Verification items for the finished model (mm, model axes). A direction names the side the tool comes from. Give positions to 0.01 mm unless a question says otherwise; leave off trailing zeros. Loops run counter-clockwise (first coordinate to the right, second up) from the corner with the lowest first, then second, coordinate; pieces in that order, holes last. Notation, with made-up numbers: M -25,4.5 L 14,4.5 A28 cw 14,43.5 Z; hole C 88,3.25 d11. An arc over 180 degrees is marked long. Use a Markdown table: item, result.
from build123d import *

# Parameters (mm, degrees)
BOSS_EXTRUDE1_DEPTH = 6.625
CUT_EXTRUDE1_DEPTH  = 13.25
SKETCH3_R           = 0.3
BOSS_EXTRUDE2_DEPTH = 4


with BuildPart() as part:
    # Sketch1 → Boss-Extrude1 (new, symmetric)
    with BuildSketch(Plane(origin=(0, 0, 0), x_dir=(0, 0, -1), z_dir=(1, 0, 0))):
        Polygon((0, 0), (0, 12.53), (14.54, 12.53), (18.15, 5), (18.15, 0), align=None)
    extrude(amount=BOSS_EXTRUDE1_DEPTH, both=True)

    # Sketch2 → Cut-Extrude1 (cut)
    with BuildSketch(Plane.XY):
        Polygon((-2.758412662, 1.863268477), (-2.758412662, 0.55), (2.758412662, 0.55), (2.758412662, 1.863268477), (3.967697722, 1.863268477), (3.967697722, 3.689249531), (5.425, 3.689249531), (5.425, 11.073209492), (3.069315997, 11.073209492), (3.069315997, 11.97), (-3.069315997, 11.97), (-3.069315997, 11.073209492), (-5.425, 11.073209492), (-5.425, 3.689249531), (-3.967697722, 3.689249531), (-3.967697722, 1.863268477), align=None)
    extrude(amount=-CUT_EXTRUDE1_DEPTH, mode=Mode.SUBTRACT)

    # Sketch3 → Boss-Extrude2 (add)
    with BuildSketch(Plane.XZ):
        with Locations(Location((2.54, -16.9, 0), (0, 0, 270))):
            Circle(SKETCH3_R)
        with Locations(Location((0, -16.9, 0), (0, 0, 270))):
            Circle(SKETCH3_R)
        with Locations(Location((-2.54, -16.9, 0), (0, 0, 270))):
            Circle(SKETCH3_R)
        with Locations(Location((0, -14.36, 0), (0, 0, 270))):
            Circle(SKETCH3_R)
        with Locations(Location((-2.54, -14.36, 0), (0, 0, 270))):
            Circle(SKETCH3_R)
        with Locations(Location((2.54, -14.36, 0), (0, 0, 270))):
            Circle(SKETCH3_R)
    extrude(amount=BOSS_EXTRUDE2_DEPTH)


solid = part.part
(1) Draft check along Y on faces 3 (the flat face through (6.625, 6, -9)), 4 (the flat face through (0, 12.53, -7)), 5 (the flat face through (-3.968, 3, -7)). Enter one of: +Y half, -Y half, draft (parallel to the pull), parting line (faces both ways), or undercut.
Results below:
| item | result |
|---|---|
| face 3 | draft |
| face 4 | +Y half |
| face 5 | undercut |
(2) Cross-section at D-D on y = 8.75. Record the cut outline in (x, z) (3 decimals).
Results below:
| item | result |
|---|---|
| outline | M -6.625,-16.352 L 6.625,-16.352 L 6.625,0 L 5.425,0 L 5.425,-13.25 L -5.425,-13.25 L -5.425,0 L -6.625,0 Z |
(3) Cross-section at C-C on x = 0. Record the cut outline in (y, z), then the cut area to 3 significant figures.
Results below:
| item | result |
|---|---|
| outline | M -4,-17.2 L 0,-17.2 L 0,-18.15 L 5,-18.15 L 12.53,-14.54 L 12.53,0 L 11.97,0 L 11.97,-13.25 L 0.55,-13.25 L 0.55,0 L 0,0 L 0,-14.06 L -4,-14.06 L -4,-14.66 L 0,-14.66 L 0,-16.6 L -4,-16.6 Z |
| area | 67.3 mm^2 |
(4) Cross-section at B-B on y = -0.5. Record the cut outline in (x, z).
Results below:
| item | result |
|---|---|
| outline | C -2.54,-16.9 d0.6; C -2.54,-14.36 d0.6; C 0,-16.9 d0.6; C 0,-14.36 d0.6; C 2.54,-16.9 d0.6; C 2.54,-14.36 d0.6 |
(5) Gauge pin test, flat end, axial feed: P1, Ø0.7, axis at x = -4, z = -5, coming from the -Y side. Record the tip position at first contact, or that the pin passes through.
Results below:
| item | result |
|---|---|
| P1 | y = 0 |
(6) Cross-section at A-A on z = -11.25. Record the cut outline in (x, y) (3 decimals).
Results below:
| item | result |
|---|---|
| outline | M -6.625,0 L 6.625,0 L 6.625,12.53 L -6.625,12.53 Z; hole M -5.425,3.689 L -3.968,3.689 L -3.968,1.863 L -2.758,1.863 L -2.758,0.55 L 2.758,0.55 L 2.758,1.863 L 3.968,1.863 L 3.968,3.689 L 5.425,3.689 L 5.425,11.073 L 3.069,11.073 L 3.069,11.97 L -3.069,11.97 L -3.069,11.073 L -5.425,11.073 Z |
(7) Set-up check for faces 1 (the flat face through (0.09, 8.82, -16.32)), 2 (the flat face through (0, 0.55, -7)): record each of +Z, -Z, +X, -X, +Y, -Y from which the full face is reachable in a straight line by a thin tool's end or side.
Results below:
| item | result |
|---|---|
| face 1 | -Z, +X, -X, +Y |
| face 2 | +Z |
(8) Material ranges on line 1 (X direction, y = 11.75, z = -8) (3 decimals); line 2 (Y direction, x = -4.75, z = -6.75); line 3 (Y direction, x = -1.75, z = -1.25), recorded low to high.
Results below:
| item | result |
|---|---|
| line 1 | -6.625 to -3.069, 3.069 to 6.625 |
| line 2 | 0 to 3.69, 11.07 to 12.53 |
| line 3 | 0 to 0.55, 11.97 to 12.53 |
